Check sheet for the modelled part. Datum: model origin and axes. Units: mm. Round coordinates to 2 decimals unless told otherwise and drop trailing zeros. Write each loop counter-clockwise with the first axis right and the second up, starting at its lowest first coordinate (ties: lowest second). Pieces come first, ordered by that corner, then holes. Notation, with made-up numbers: (59.5, 3.5) -> (101.5, 3.5) arc R15 ccw to (101.5, 22.5) -> close; hole circle Ø4 at (82, -13). An arc over 180 degrees is marked (long way). One line per item, written item: value. Start each with the question number.
Autodesk Inventor part; units mm, degrees
ref_plane "YZ Plane" through (0, 0, 0) normal (1, 0, 0) x (0, 1, 0)
ref_plane "XZ Plane" through (0, 0, 0) normal (0, 1, 0) x (-1, 0, 0)
ref_plane "XY Plane" through (0, 0, 0) normal (0, 0, 1) x (1, 0, 0)
sketch "Sketch1" plane through (0, 0, 0) normal (0, 1, 0) x (-1, 0, 0)
  line L0 (349.8743, 0) -> (258.4057, -158.4282)
  line L1 (174.9371, -303) -> (-174.9371, -303)
  line L2 (-174.9371, -303) -> (-349.8743, 0)
  line L3 (-349.8743, 0) -> (-174.9371, 303)
  line L4 (-174.9371, 303) -> (174.9371, 303)
  line L5 (258.4057, 158.4282) -> (349.8743, 0)
  line L6 (0, 0) -> (-8, 0)
  line L7 (-8, 0) -> (-8, -303)
  line L8 (-8, -303) -> (8, -303)
  line L9 (8, -303) -> (8, 0)
  line L10 (8, 0) -> (-8, 0)
  circle A0 centre (0, 0) radius 2.5
  line L11 (258.4057, 158.4282) -> (-4, 6.9282)
  line L12 (4, -6.9282) -> (266.4057, 144.5718)
  line L13 (-4, 6.9282) -> (4, -6.9282)
  line L14 (-266.4057, 144.5718) -> (-4, -6.9282)
  line L15 (4, 6.9282) -> (-258.4057, 158.4282)
  line L16 (-4, -6.9282) -> (4, 6.9282)
  line L17 (8, -4.6188) -> (8, -151.5)
  line L18 (8, -151.5) -> (-8, -151.5)
  line L19 (-8, -151.5) -> (-8, -303)
  line L20 (-8, -4.6188) -> (-4, -6.9282)
  line L21 (4, -6.9282) -> (-4, -6.9282)
  line L22 (-266.4057, 144.5718) -> (-258.4057, 158.4282)
  line L23 (-127.2028, 82.6782) -> (-135.2028, 68.8218)
  line L24 (-135.2028, 68.8218) -> (-8, -4.6188)
  line L25 (-266.4057, 144.5718) -> (-349.8743, 0)
  line L26 (-174.9371, -303) -> (-349.8743, 0)
  line L27 (-174.9371, -303) -> (-8, -303)
  line L28 (0, 9.2376) -> (8, 0)
  dimension "d0" = 303
  dimension "d1" = 303
  dimension "d2" = 8
  dimension "d3" = 16
  dimension "d4" = 5
  dimension "d7" = 360
extrude "Extrusion1" add sketch "Sketch1" along normal blind 3 contours L1 L7 L18 L9 | L1 L2 L3 L14 L7 | L18 L7 L14 L21 L12 L9 | L12 L13 A0 L10 L9 | L14 L23 L15 L11 L13 A0 L6 L7 | L7 L6 A0 L16 L14 | L10 A0 L16 L28 | L21 L16 A0 L13 | L3 L15 L23 L14 | A0 L13 L10 | L10 L16 A0 | L28 L15 L16 | L16 A0 L13 L11 L28 | A0 L16 L13 | A0 L13 L6 | L6 L16 A0 | L13 A0 L16
sketch "Sketch2" plane through (0, 3, 0) normal (0, 1, 0) x (1, 0, 0)
  line L0 (-8, 303) -> (-8, 0)
  line L1 (-8, 0) -> (-8, 151.5)
  line L2 (-8, 151.5) -> (8, 151.5)
  line L3 (8, 151.5) -> (8, 0)
  line L4 (8, 0) -> (-8, 0)
  line L5 (0, -9.2376) -> (258.4057, -158.4282)
  line L6 (258.4057, -158.4282) -> (126.3368, -82.1782)
  line L7 (126.3368, -82.1782) -> (134.8368, -67.4558)
  line L8 (134.8368, -67.4558) -> (266.9057, -143.7058)
  line L9 (266.9057, -143.7058) -> (258.4057, -158.4282)
  point P0 (0, 0)
  dimension "d11" = 151.5
  dimension "d12" = 16
  dimension "d13" = 152.5
  dimension "d14" = 17
extrude "Extrusion2" cut sketch "Sketch2" against normal blind 3
sketch "Sketch3" plane through (0, 3, 0) normal (0, 1, 0) x (1, 0, 0)
  line L0 (174.9371, 303) -> (-8, 303)
  line L1 (174.9371, 303) -> (139.9371, 303)
  line L2 (139.9371, 303) -> (139.9371, 295)
  line L3 (139.9371, 295) -> (174.9371, 295)
  line L4 (174.9371, 295) -> (174.9371, 303)
  line L5 (349.8743, 0) -> (174.9371, 303)
  line L6 (174.9371, 303) -> (192.4371, 272.6891)
  line L7 (192.4371, 272.6891) -> (185.5089, 268.6891)
  line L8 (185.5089, 268.6891) -> (168.0089, 299)
  line L9 (168.0089, 299) -> (174.9371, 303)
  line L10 (349.8743, 0) -> (332.3743, 30.3109)
  line L11 (332.3743, 30.3109) -> (325.4461, 26.3109)
  line L12 (325.4461, 26.3109) -> (342.9461, -4)
  line L13 (342.9461, -4) -> (349.8743, 0)
  line L14 (349.8743, 0) -> (332.3743, -30.3109)
  line L15 (332.3743, -30.3109) -> (325.4461, -26.3109)
  line L16 (325.4461, -26.3109) -> (342.9461, 4)
  line L17 (342.9461, 4) -> (349.8743, 0)
  line L18 (349.8743, 0) -> (266.9057, -143.7058)
  line L19 (349.8743, 0) -> (384.8743, 0) construction
  point P0 (0, 0)
  dimension "d17" = 35
  dimension "d18" = 8
  dimension "d19" = 35
  dimension "d20" = 8
  dimension "d21" = 35
  dimension "d22" = 8
  dimension "d23" = 35
  dimension "d24" = 120
  dimension "d25" = 8
extrude "Extrusion3" cut sketch "Sketch3" against normal blind 3
sketch "Sketch4" plane through (0, 3, 0) normal (0, 1, 0) x (1, 0, 0)
  line L0 (-54.0368, 51.4054) -> (71.5368, -21.0946)
  line L1 (71.5368, -21.0946) -> (54.0368, -51.4054)
  line L2 (54.0368, -51.4054) -> (-71.5368, 21.0946)
  line L3 (-71.5368, 21.0946) -> (-54.0368, 51.4054)
  line L4 (-54.0368, 51.4054) -> (54.0368, -51.4054) construction
  line L5 (71.5368, -21.0946) -> (-71.5368, 21.0946) construction
  line L6 (-54.0368, 51.4054) -> (90.9632, 51.4054) construction
  line L7 (-17.5, -72.5) -> (-17.5, 72.5)
  line L8 (-17.5, 72.5) -> (17.5, 72.5)
  line L9 (17.5, 72.5) -> (17.5, -72.5)
  line L10 (17.5, -72.5) -> (-17.5, -72.5)
  line L11 (-17.5, -72.5) -> (17.5, 72.5) construction
  line L12 (-17.5, 72.5) -> (17.5, -72.5) construction
  line L13 (-8, 0) -> (8, 0)
  line L14 (-17.5, -72.5) -> (127.5, -72.5) construction
  point P0 (0, 0)
  dimension "d28" = 145
  dimension "d29" = 30
  dimension "d30" = 35
  dimension "d31" = 145
  dimension "d32" = 90
  dimension "d33" = 35
extrude "Extrusion4" cut sketch "Sketch4" against normal blind 3
sketch "Sketch5" plane through (0, 3, 0) normal (0, 1, 0) x (1, 0, 0)
  line L0 (-1, 151.5) -> (-1, 191.5)
  circle A0 centre (-1, 191.5) radius 2.75
  circle A1 centre (-1, 231.5) radius 2.75
  circle A2 centre (-1, 271.5) radius 2.75
  circle A3 centre (0, 0) radius 0.5
  line L1 (126.3368, -82.1782) -> (134.8368, -67.4558)
  line L2 (126.3368, -82.1782) -> (129.5868, -76.549)
  line L3 (129.5868, -76.549) -> (103.6061, -61.549)
  line L4 (103.6061, -61.549) -> (77.6253, -46.549)
  circle A4 centre (103.6061, -61.549) radius 2.75
  circle A5 centre (77.6253, -46.549) radius 2.75
  line L5 (-8, 303) -> (-8, 151.5)
  dimension "d36" = 40
  dimension "d37" = 5.5
  dimension "d40" = 40
  dimension "d45" = 1
  dimension "d46" = 6.5
  dimension "d47" = 30
  dimension "d48" = 30
  dimension "d49" = 5.5
  dimension "d50" = 5.5
  dimension "d53" = 7
extrude "Extrusion5" cut sketch "Sketch5" against normal blind 3 contours A0 | A1 | A2 | A4 L4 L3 | A5 | L3 L4 A4
sketch "Sketch6" plane through (0, 3, 0) normal (0, 1, 0) x (1, 0, 0)
  line L0 (-8, 303) -> (-8, 151.5)
  line L1 (-8, 303) -> (344, 303)
  line L2 (344, 303) -> (344, -147)
  line L3 (344, -147) -> (-8, -147)
  line L4 (-8, -147) -> (-8, 303)
  point P0 (0, 0)
  dimension "d54" = 352
  dimension "d55" = 450
sketch "Sketch7" plane through (0, 3, 0) normal (0, 1, 0) x (1, 0, 0)
  line L0 (139.9371, 303) -> (-8, 303)
  line L1 (-8, 303) -> (343, 303)
  line L2 (343, 303) -> (343, -144)
  line L3 (343, -144) -> (-8, -144)
  line L4 (-8, -144) -> (-8, 303)
  point P0 (0, 0)
  dimension "d56" = 351
  dimension "d57" = 447
fillet "Fillet1" radius 10 2 edges at (340.6367, 1.5, 0) (170.3183, 1.5, -295)
properties part number "Acrylic_bottom"
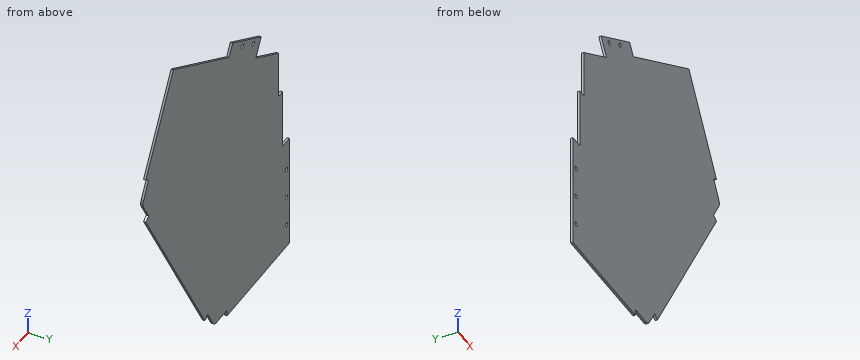
1. Cross-section at A-A (y = 1.4). Record the cut outline in (x, z), plus the area to 3 significant figures.
2. Cross-section at C-C (z = -200.5). Record the cut outline in (x, y).
3. Material ranges on probe 1 along Z at (x, y) = (-1, 0.85); probe 2 along X at (y, z) = (1, -271.5); probe 3 along X at (y, z) = (0.75, -191.5), recorded low to high.
4. Cross-section at B-B (x = 228.5). Record the cut outline in (y, z).
5. Depth check by flat-ended pin: pin 1 Ø7 at (x, z) = (77.63, 46.55) entering from +Y; pin 2 Ø1.5 at (x, y) = (155, 1) entering from -Z; pin 3 Ø1.5 at (x, y) = (14, 2) entering from +Z; pin 4 Ø0.9 at (y, z) = (1, -107.5) entering from -X. Enter the tip coordinate at first touch or a pass-through.
Working result:
1. outline: (-8, -303) -> (139.94, -303) -> (139.94, -295) -> (164.54, -295) arc R10 ccw to (173.21, -290) -> (185.51, -268.69) -> (192.44, -272.69) -> (332.37, -30.31) -> (325.45, -26.31) -> (337.75, -5) arc R10 ccw to (337.75, 5) -> (325.45, 26.31) -> (332.37, 30.31) -> (266.91, 143.71) -> (134.84, 67.46) -> (126.34, 82.18) -> (58.79, 43.18) -> (71.54, 21.09) -> (17.5, -10.1) -> (17.5, -72.5) -> (8, -72.5) -> (8, -151.5) -> (-8, -151.5) -> close; hole circle Ø5.5 at (-1, -271.5); hole circle Ø5.5 at (-1, -231.5); hole circle Ø5.5 at (-1, -191.5); hole circle Ø5.5 at (77.63, 46.55); hole circle Ø5.5 at (103.61, 61.55)
1. area: 102,000 mm^2
2. outline: (-8, 0) -> (234.12, 0) -> (234.12, 3) -> (-8, 3) -> close
3. probe 1: z = -303 to -274.25, -268.75 to -234.25, -228.75 to -194.25, -188.75 to -151.5
3. probe 2: x = -8 to -3.75, 1.75 to 183.89, 190.38 to 193.12
3. probe 3: x = -8 to -3.75, 1.75 to 239.31
4. outline: (0, -210.23) -> (3, -210.23) -> (3, 121.53) -> (0, 121.53) -> close
5. pin 1: stops at y = 3
5. pin 2: stops at z = -295
5. pin 3: stops at z = -72.5
5. pin 4: stops at x = 8
